```python
from build123d import *

# Parameters (mm, degrees)
SKETCH1_W           = 3
SKETCH1_H           = 3
SKETCH1_W_2         = 14
SKETCH1_H_2         = 10
BOSS_EXTRUDE1_DEPTH = 3


with BuildPart() as part:
    # Sketch1 → Boss-Extrude1 (new body)
    with BuildSketch(Plane(origin=(0, 0, 0), x_dir=(1, 0, 0), z_dir=(0, 1, 0))):
        Polygon((-2.229716691, 32.311583722), (-23.229716691, 32.311583722), (-23.229716691, 22.311583722), (7.770283309, 22.311583722), (7.770283309, 57.311583722), (-23.229716691, 57.311583722), (-23.229716691, 47.311583722), (-2.229716691, 47.311583722), align=None)
        with Locations((-21.729716691, 39.811583722)):
            Rectangle(SKETCH1_W, SKETCH1_H)
        Polygon((-23.229716691, 32.311583722), (-23.229716691, 34.311583722), (-23.229716691, 38.311583722), (-33.229716691, 38.311583722), (-33.229716691, 32.311583722), (-33.229716691, 22.311583722), (-23.229716691, 22.311583722), align=None)
        Polygon((-33.229716691, 38.311583722), (-23.229716691, 38.311583722), (-23.229716691, 41.311583722), (-23.229716691, 45.311583722), (-23.229716691, 47.311583722), (-23.229716691, 57.311583722), (-33.229716691, 57.311583722), (-33.229716691, 47.311583722), align=None)
        with Locations((-40.229716691, 52.311583722)):
            Rectangle(SKETCH1_W_2, SKETCH1_H_2)
        with Locations((-40.229716691, 27.311583722)):
            Rectangle(SKETCH1_W_2, SKETCH1_H_2)
        Polygon((-47.229716691, 22.311583722), (-47.229716691, 32.311583722), (-47.229716691, 34.311583722), (-47.229716691, 38.311583722), (-57.229716691, 38.311583722), (-57.229716691, 22.311583722), align=None)
        Polygon((-47.229716691, 45.311583722), (-47.229716691, 47.311583722), (-47.229716691, 57.311583722), (-57.229716691, 57.311583722), (-57.229716691, 38.311583722), (-47.229716691, 38.311583722), (-47.229716691, 41.311583722), align=None)
        with Locations((-45.729716691, 39.811583722)):
            Rectangle(SKETCH1_W, SKETCH1_H)
    extrude(amount=BOSS_EXTRUDE1_DEPTH)


solid = part.part
```
The model under review builds one solid part; all positions refer to its coordinate system, in mm. A direction names the side the tool comes from. Round coordinates to 2 decimals unless told otherwise and drop trailing zeros. Loops run counter-clockwise (first coordinate to the right, second up) from the corner with the lowest first, then second, coordinate; pieces in that order, holes last.
1) Tool access review of faces 1 (the face through (-22, 1, -38.312)), 2 (the face through (-25, 1, -22.312)): name each direction out of +Z, -Z, +X, -X, +Y, -Y from which nothing blocks a thin tool from reaching the whole face with its end or side.
Values follow:
face 1: +Y, -Y
face 2: +Z, +X, -X, +Y, -Y
2) Consider section D-D on y = 0.45. State the section outline as (x, z) points.
Values follow:
outline: (-57.23, -57.31) - (7.77, -57.31) - (7.77, -22.31) - (-57.23, -22.31) - close; hole (-47.23, -47.31) - (-33.23, -47.31) - (-33.23, -32.31) - (-47.23, -32.31) - (-47.23, -38.31) - (-44.23, -38.31) - (-44.23, -41.31) - (-47.23, -41.31) - close; hole (-23.23, -47.31) - (-2.23, -47.31) - (-2.23, -32.31) - (-23.23, -32.31) - (-23.23, -38.31) - (-20.23, -38.31) - (-20.23, -41.31) - (-23.23, -41.31) - close
3) Wall thickness on line 1 along X through (y, z) = (0.45, -33.5); line 2 along X through (y, z) = (2.35, -39); line 3 along Z through (x, y) = (-21, 2.35): over which ranges is each line inside the solid? List them lowest first.
Values follow:
line 1: x = -57.23 to -47.23, -33.23 to -23.23, -2.23 to 7.77
line 2: x = -57.23 to -44.23, -33.23 to -20.23, -2.23 to 7.77
line 3: z = -57.31 to -47.31, -41.31 to -38.31, -32.31 to -22.31
4) Consider section B-B on x = -22.5. State the section outline as (y, z) points, then the cut area to 3 significant figures.
Values follow:
outline: (0, -57.31) - (3, -57.31) - (3, -47.31) - (0, -47.31) - close; (0, -41.31) - (3, -41.31) - (3, -38.31) - (0, -38.31) - close; (0, -32.31) - (3, -32.31) - (3, -22.31) - (0, -22.31) - close
area: 69.0 mm2
5) Consider section C-C on x = -16. State the section outline as (y, z) points, then the cut area to 3 significant figures.
Values follow:
outline: (0, -57.31) - (3, -57.31) - (3, -47.31) - (0, -47.31) - close; (0, -32.31) - (3, -32.31) - (3, -22.31) - (0, -22.31) - close
area: 60.0 mm2
6) Consider section A-A on z = -34.5. State the section outline as (x, y) points, then the cut area to 3 significant figures.
Values follow:
outline: (-57.23, 0) - (-47.23, 0) - (-47.23, 3) - (-57.23, 3) - close; (-33.23, 0) - (-23.23, 0) - (-23.23, 3) - (-33.23, 3) - close; (-2.23, 0) - (7.77, 0) - (7.77, 3) - (-2.23, 3) - close
area: 90.0 mm2
7) The part is to be moulded in two halves that separate along X. For faces 3 (the face through (7.77, 1, -40)), 4 (the face through (-47.23, 1, -44)), 5 (the face through (-40, 1, -32.312)), 6 (the face through (-25, 0, -40)), say which applies: pulls with the +X half, pulls with the -X half, needs draft (parallel to the pull), parting line crosses it, or undercut.
Values follow:
face 3: pulls with the +X half
face 4: undercut
face 5: undercut
face 6: needs draft
8) Clearance check with a flat-ended pin moving along its axis: P1, Ø1.5, axis at x = -14.5, z = -28.5, coming from the -Y side. State where the tip first meets the part, or that it passes through.
Values follow:
P1: stops at y = 0
